from build123d import *

# Parameters (mm, degrees)
SKETCH1_W           = 7
SKETCH1_H           = 3
BOSS_EXTRUDE1_DEPTH = 1.5
SKETCH2_W           = 9
SKETCH2_H           = 5
BOSS_EXTRUDE2_DEPTH = 1
SKETCH3_R           = 0.75
BOSS_EXTRUDE3_DEPTH = 0.25


with BuildPart() as part:
    # Sketch1 → Boss-Extrude1 (new body)
    with BuildSketch(Plane(origin=(0, 0, 0), x_dir=(1, 0, 0), z_dir=(0, 1, 0))):
        Rectangle(SKETCH1_W, SKETCH1_H)
    extrude(amount=BOSS_EXTRUDE1_DEPTH)

    # Sketch2 → Boss-Extrude2 (add)
    with BuildSketch(Plane.XZ):
        Rectangle(SKETCH2_W, SKETCH2_H)
    extrude(amount=BOSS_EXTRUDE2_DEPTH)

    # Sketch3 → Boss-Extrude3 (add, symmetric)
    with BuildSketch(Plane.XY):
        Polygon((-1.5, 1.5), (-1.5, 2.5), (-2, 2.5), (-2, 7.5), (-1, 8.5), (1, 8.5), (2, 7.5), (2, 1.936391511), (1.5, 1.936391511), (1.5, 1.5), align=None)
        with Locations((0, 6)):
            Circle(SKETCH3_R, mode=Mode.SUBTRACT)
    extrude(amount=BOSS_EXTRUDE3_DEPTH, both=True)


solid = part.part
The listing builds one solid part. Answer for the finished solid, in the listing's coordinates (mm). A direction names the side the tool comes from. Coordinates: 2 decimals unless noted, no trailing zeros. Write each loop counter-clockwise with the first axis right and the second up, starting at its lowest first coordinate (ties: lowest second). Pieces come first, ordered by that corner, then holes. Notation, with made-up numbers: M 31.5,55 L 57.5,55 A16 cw 57.5,74 Z; hole C -17.75,20.25 d8. An arc over 180 degrees is marked long. Use one line per item in the form item = value.
Item 1: Given P1, Ø2.5, axis at x = 0, y = 6, coming from the +Z side; P2, Ø1.2, axis at x = -0.5, y = 3.5, coming from the -Z side; P3, Ø0.8, axis at x = -1, y = 0.5, coming from the +Z side, each flat-ended and moving along its own axis, determine where each tip first touches the part or whether it passes through.
Model answer:
P1 = 0.25
P2 = -0.25
P3 = 1.5
Item 2: For faces 1 (the face through (0, 1, 1.5)), 2 (the face through (-0.1, -0.5, 2.5)), 3 (the face through (1.5, 8, 0)), 4 (the face through (-3.5, 1, 0)), 5 (the face through (0, 5, -0.25)), determine the directions among +Z, -Z, +X, -X, +Y, -Y from which every point of the face is accessible in a straight line to the end or side of a thin tool.
Model answer:
face_1 = +Z, +X, -X, +Y
face_2 = +Z, +X, -X, +Y, -Y
face_3 = +Z, -Z, +X, +Y
face_4 = +Z, -Z, -X, +Y
face_5 = -Z, +X, -X, +Y
Item 3: Find section B-B, the plane y = 6. Give the vertices of the cut face in (x, z), plus the area to 3 significant figures.
Model answer:
outline = M -2,-0.25 L -0.75,-0.25 L -0.75,0.25 L -2,0.25 Z; M 0.75,-0.25 L 2,-0.25 L 2,0.25 L 0.75,0.25 Z
area = 1.25 mm2
Item 4: Find section C-C, the plane z = 0.1. Give the vertices of the cut face in (x, y), plus the area to 3 significant figures.
Model answer:
outline = M -4.5,-1 L 4.5,-1 L 4.5,0 L 3.5,0 L 3.5,1.5 L 1.5,1.5 L 1.5,1.94 L 2,1.94 L 2,7.5 L 1,8.5 L -1,8.5 L -2,7.5 L -2,2.5 L -1.5,2.5 L -1.5,1.5 L -3.5,1.5 L -3.5,0 L -4.5,0 Z; hole C 0,6 d1.5
area = 44.0 mm2
Item 5: Find the intervals of material crossed by probe 1 along Y at (x, z) = (0, 0.1); probe 2 along Y at (x, z) = (2.5, -0.9); probe 3 along Z at (x, y) = (-0.75, 3.75), in increasing order.
Model answer:
probe_1 = -1 to 5.25, 6.75 to 8.5
probe_2 = -1 to 1.5
probe_3 = -0.25 to 0.25
Item 6: Find section A-A, the plane x = 0. Give the vertices of the cut face in (y, z), plus the area to 4 significant figures.
Model answer:
outline = M -1,-2.5 L 0,-2.5 L 0,-1.5 L 1.5,-1.5 L 1.5,-0.25 L 5.25,-0.25 L 5.25,0.25 L 1.5,0.25 L 1.5,1.5 L 0,1.5 L 0,2.5 L -1,2.5 Z; M 6.75,-0.25 L 8.5,-0.25 L 8.5,0.25 L 6.75,0.25 Z
area = 12.25 mm2
Item 7: Find section D-D, the plane z = -0.5. Give the vertices of the cut face in (x, y).
Model answer:
outline = M -4.5,-1 L 4.5,-1 L 4.5,0 L 3.5,0 L 3.5,1.5 L -3.5,1.5 L -3.5,0 L -4.5,0 Z
Item 8: The mould has two halves that part along X. Classify faces 6 (the face through (-4.5, -0.5, 0)), 7 (the face through (-0.163, 5.268, -0.004)), 8 (the face through (3.5, 1, 0)): released by +X, released by -X, zero draft, split by the parting line, or undercut.
Model answer:
face_6 = released by -X
face_7 = undercut
face_8 = released by +X
